The figure shows three views and two pictorial views of one solid part (mm, origin at its lowest corner). Answer the questions. A direction names the side the tool comes from. Coordinates: 2 decimals unless noted, no trailing zeros. Loops run counter-clockwise (first coordinate to the right, second up) from the corner with the lowest first, then second, coordinate; pieces in that order, holes last. Notation, with made-up numbers: M 28.5,-24.75 L 86.5,-24.75 A30 cw 86.5,13.25 Z; hole C 83,-13 d6. An arc over 180 degrees is marked long. Answer in a Markdown table with one row per item. Add a question column.
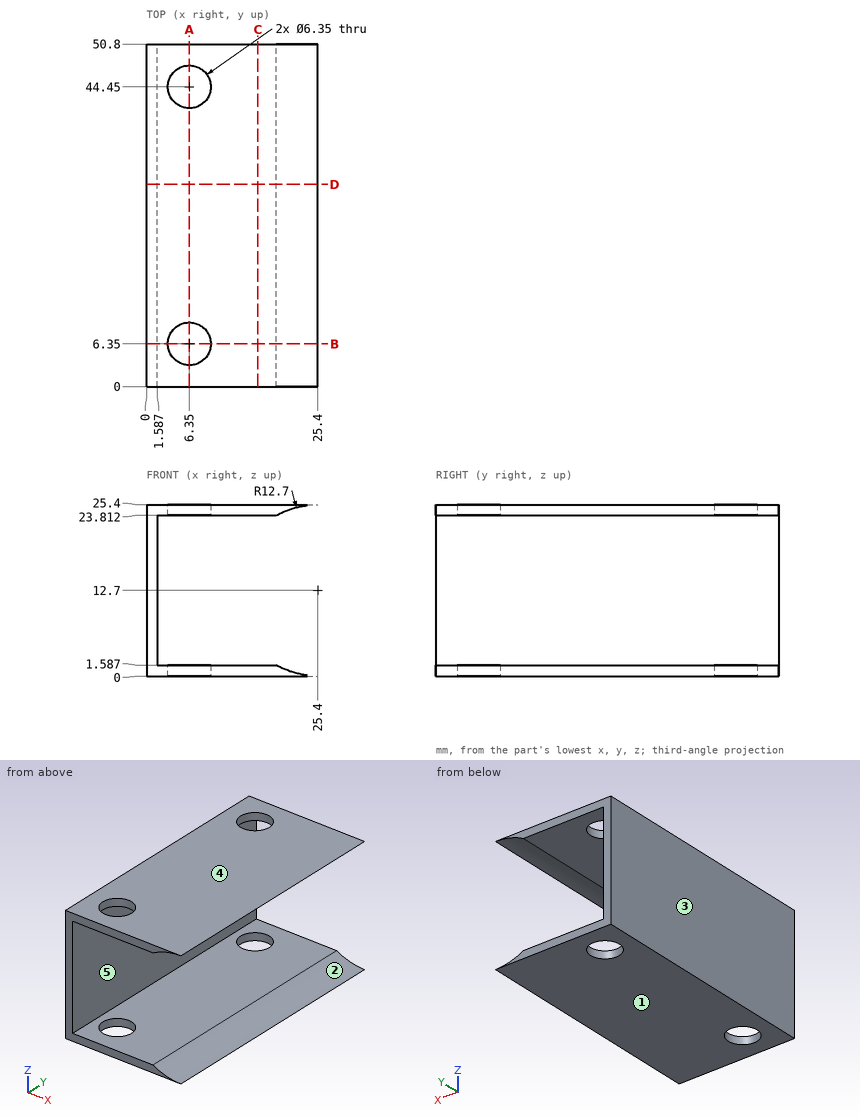
(1) Each of these flat-tipped pins is pushed along its axis until it touches: pin 1 (7.5 mm diameter, centred on x = 6.35, y = 6.35, fed in from -Z); pin 2 (5.5 mm diameter, centred on x = 6.35, y = 44.45, fed in from -Z); pin 3 (6 mm diameter, centred on y = 27.5, z = 7.5, fed in from +X). Where does it stop, or does it pass through?
(2) A cutting plane is placed at C-C (x = 16.5). Give the vertices of the cut face in (y, z).
(3) For the marked faces 4 and 5, determine the directions among +Z, -Z, +X, -X, +Y, -Y from which every point of the face is accessible in a straight line to the end or side of a thin tool.
(4) A cutting plane is placed at D-D (y = 30). Give the vertices of the cut face in (x, z).
(5) A cutting plane is placed at A-A (x = 6.35). Give the vertices of the cut face in (y, z) (1 decimal), plus the area to 3 significant figures.
(6) A cutting plane is placed at B-B (y = 6.35). Give the vertices of the cut face in (x, z) (1 decimal).
(7) Straight lines are drawn through the part: line 1 (Y direction, x = 6.35, z = 24.75) (1 decimal); line 2 (Z direction, x = 4.5, y = 18.5); line 3 (X direction, y = 38, z = 3.75). For each, find the intervals that lie inside material, in ascending order.
(8) The mould has two halves that part along Z. Classify the marked faces 1, 2 and 3: released by +Z, released by -Z, zero draft, split by the parting line, or undercut.
Solved:
| question | item | result |
|---|---|---|
| 1 | pin 1 | stops at z = 0 |
| 1 | pin 2 | passes through |
| 1 | pin 3 | stops at x = 1.59 |
| 2 | outline | M 0,0 L 50.8,0 L 50.8,1.59 L 0,1.59 Z; M 0,23.81 L 50.8,23.81 L 50.8,25.4 L 0,25.4 Z |
| 3 | face 4 | +Z, +X, -X, +Y, -Y |
| 3 | face 5 | +X, +Y, -Y |
| 4 | outline | M 0,0 L 25.4,0 A12.7 cw 19.25,1.59 L 1.59,1.59 L 1.59,23.81 L 19.25,23.81 A12.7 cw 25.4,25.4 L 0,25.4 Z |
| 5 | outline | M 0,0 L 3.2,0 L 3.2,1.6 L 0,1.6 Z; M 0,23.8 L 3.2,23.8 L 3.2,25.4 L 0,25.4 Z; M 9.5,0 L 41.3,0 L 41.3,1.6 L 9.5,1.6 Z; M 9.5,23.8 L 41.3,23.8 L 41.3,25.4 L 9.5,25.4 Z; M 47.6,0 L 50.8,0 L 50.8,1.6 L 47.6,1.6 Z; M 47.6,23.8 L 50.8,23.8 L 50.8,25.4 L 47.6,25.4 Z |
| 5 | area | 121 mm² |
| 6 | outline | M 0,0 L 3.2,0 L 3.2,1.6 L 1.6,1.6 L 1.6,23.8 L 3.2,23.8 L 3.2,25.4 L 0,25.4 Z; M 9.5,0 L 25.4,0 A12.7 cw 19.3,1.6 L 9.5,1.6 Z; M 9.5,23.8 L 19.3,23.8 A12.7 cw 25.4,25.4 L 9.5,25.4 Z |
| 7 | line 1 | y = 0 to 3.2, 9.5 to 41.3, 47.6 to 50.8 |
| 7 | line 2 | z = 0 to 1.59, 23.81 to 25.4 |
| 7 | line 3 | x = 0 to 1.59 |
| 8 | face 1 | released by -Z |
| 8 | face 2 | undercut |
| 8 | face 3 | zero draft |
